from build123d import *

# Parameters (mm, degrees)
F0_R     = 6.35
F1_DEPTH = 4.7625
F2_SIZE  = 0.762


# Not quite as in the source:
# - a feature names something its author has since deleted; it is built from what else it names


with BuildPart() as f1:
    # F0 (on Front) → F1 (new body, symmetric)
    with BuildSketch(Plane.XZ):
        Polygon((7.3323484187, 12.7), (-7.3323484187, 12.7), (-14.6646968374, 0), (-7.3323484187, -12.7), (7.3323484187, -12.7), (14.6646968374, 0), align=None)
        Circle(F0_R, mode=Mode.SUBTRACT)
    extrude(amount=F1_DEPTH, both=True)

    # F2
    f2_edges = [f1.edges().sort_by_distance(p)[0] for p in [
        (-6.35, -4.7625, 0),
        (-6.35, 4.7625, 0),
    ]]
    chamfer(f2_edges, length=F2_SIZE)

    # F4: sweep along a path in F4_path
    with BuildLine(Plane(origin=(7.112, -4.7625, 0), x_dir=(0, 0, -1), z_dir=(0, 1, 0))) as f4_path:
        CenterArc((0, 7.112), 7.112, 0, 360)
    # F3 (on Top) → F4 (sweep, cut)
    with BuildSketch(Plane.XY):
        Polygon((-14.8424788945, -5.049383917), (-12.7, -4.7852232567), (-14.8424788945, -3.5482624902), align=None)
    sweep(path=f4_path.line, mode=Mode.SUBTRACT)


solid = f1.part
Part model, mm, in its own coordinate system. Round coordinates to 2 decimals unless told otherwise and drop trailing zeros. Order: outer loops, then holes, each group sorted by start corner. A loop starts at its lowest first (then second) coordinate and runs counter-clockwise, first axis right, second up. Notation, with made-up numbers: (34.5, -5.5) -> (50.5, -5.5) arc R15 ccw to (50.5, 0.5) -> close; hole circle Ø9 at (13, -33.5). An arc over 180 degrees is marked (long way). Put each result on its own line as item: value.
Q1. Pull direction X, two halves, no side cores. Call faces 1 (the face through (-6.627, -4.492, 11.424)), 2 (the face through (-1.38, 0.06, -6.2)), 3 (the face through (13.21, -4.49, 0.03)), 4 (the face through (0, 0, -12.7)): pulls with the +X half, pulls with the -X half, needs draft (parallel to the pull), parting line crosses it, or undercut.
From the geometry:
face 1: pulls with the -X half
face 2: undercut
face 3: pulls with the +X half
face 4: needs draft
Q2. Band-saw the part on B-B (y = 1). Give the cut face in (x, z), and give its area (3 significant figures).
From the geometry:
outline: (-14.66, 0) -> (-7.33, -12.7) -> (7.33, -12.7) -> (14.66, 0) -> (7.33, 12.7) -> (-7.33, 12.7) -> close; hole circle Ø12.7 at (0, 0)
area: 432 mm2
Q3. Wall check: line 1 (Z direction, x = 0, y = 2.25); line 2 (Z direction, x = 11, y = -4); line 3 (X direction, y = 0.5, z = -5.5). Give the ranges that are in metal, low to high. Write a range as [from, to].
From the geometry:
line 1: z = [-12.7, -6.35], [6.35, 12.7]
line 2: z = [-6.35, 6.35]
line 3: x = [-11.49, -3.17], [3.17, 11.49]
Q4. Pin check, flat tips, straight feed: pin 1 Ø3 at (y, z) = (-0.5, 7.5) entering from -X; pin 2 Ø2 at (x, z) = (-2, 3) entering from +Y; pin 3 Ø1 at (y, z) = (3.5, -1) entering from +X. Stop position of each tip, or through.
From the geometry:
pin 1: stops at x = -11.2
pin 2: passes through
pin 3: stops at x = 14.38
Q5. Band-saw the part on A-A (x = 0). Give the cut face in (y, z), and give its area (3 significant figures).
From the geometry:
outline: (-4.76, -12.7) -> (4.76, -12.7) -> (4.76, -7.11) -> (4, -6.35) -> (-4, -6.35) -> (-4.76, -7.11) -> close; (-4.76, 7.11) -> (-4, 6.35) -> (4, 6.35) -> (4.76, 7.11) -> (4.76, 12.7) -> (-4.76, 12.7) -> close
area: 120 mm2
